Input: part model. Units: mm. Frame: model coordinates. A direction names the side the tool comes from. Give positions to 0.01 mm unless a question says otherwise; leave off trailing zeros. Loops run counter-clockwise (first coordinate to the right, second up) from the corner with the lowest first, then second, coordinate; pieces in that order, holes last. Notation, with made-up numbers: M 31,40 L 64,40 A21 ccw 64,50 Z; hole C 80,-29.5 d2. An arc over 180 degrees is marked long. Use a Markdown table: item, result. Add a question column.
from build123d import *

# Parameters (mm, degrees)
SKETCH1_R               = 1.05
SKETCH1_R_2             = 4.95
BOSS_EXTRUDE1_DEPTH     = 1.5
CIRPATTERN1_COUNT       = 14
SKETCH2_R               = 3.5
SKETCH2_R_2             = 2
SKETCH2_W               = 2
SKETCH2_H               = 4
SKETCH2_W_2             = 4
SKETCH2_H_2             = 2
BOSS_EXTRUDE2_DEPTH     = 7.5
SKETCH3_R               = 2
CUT_EXTRUDE1_DEPTH      = 0.1
SKETCH4_R               = 1
CUT_EXTRUDE2_DEPTH      = 1
CUT_EXTRUDE3_DEPTH      = 1
CUT_EXTRUDE3_DEPTH_BACK = 10


with BuildPart() as part:
    # Sketch1 → Boss-Extrude1 (new body)
    with BuildSketch(Plane(origin=(0, 0, 0), x_dir=(1, 0, 0), z_dir=(0, 1, 0))):
        with Locations((0, 4.95)):
            Circle(SKETCH1_R)
        Circle(SKETCH1_R_2)
    boss_extrude1 = extrude(amount=BOSS_EXTRUDE1_DEPTH)

    # CirPattern1: Boss-Extrude1 ×14 about axis
    cirpattern1_axis = Axis((0, 0, 0), (0, 1, 0))
    for i in range(1, CIRPATTERN1_COUNT):
        add(boss_extrude1.rotate(cirpattern1_axis, i * 360 / CIRPATTERN1_COUNT))

    # Sketch2 → Boss-Extrude2 (add)
    with BuildSketch(Plane(origin=(0, 1.5, 0), x_dir=(1, 0, 0), z_dir=(0, 1, 0))):
        Circle(SKETCH2_R)
        Circle(SKETCH2_R_2, mode=Mode.SUBTRACT)
        Rectangle(SKETCH2_W, SKETCH2_H, mode=Mode.SUBTRACT)
        Rectangle(SKETCH2_W_2, SKETCH2_H_2, mode=Mode.SUBTRACT)
        with BuildLine():
            ThreePointArc((-1, 1.732050808), (-0.517638086, 1.931851654), (9e-09, 2))
            Line((9e-09, 2), (-1, 2))
            Line((-1, 2), (-1, 1.732050808))
        make_face()
        with BuildLine():
            Line((1, 1.732050808), (1, 2))
            Line((1, 2), (9e-09, 2))
            ThreePointArc((9e-09, 2), (0.517638095, 1.931851651), (1, 1.732050808))
        make_face()
        with BuildLine():
            Line((2, 1), (1.732050808, 1))
            ThreePointArc((1.732050808, 1), (1.931851653, 0.51763809), (2, 0))
            Line((2, 0), (2, 1))
        make_face()
        with BuildLine():
            ThreePointArc((1.732050808, 1), (1.414213562, 1.414213562), (1, 1.732050808))
            Line((1, 1.732050808), (1, 1))
            Line((1, 1), (1.732050808, 1))
        make_face()
        with BuildLine():
            Line((-1, 1), (-1, 1.732050808))
            ThreePointArc((-1, 1.732050808), (-1.414213562, 1.414213562), (-1.732050808, 1))
            Line((-1.732050808, 1), (-1, 1))
        make_face()
        with BuildLine():
            ThreePointArc((-2, 0), (-1.931851653, 0.51763809), (-1.732050808, 1))
            Line((-1.732050808, 1), (-2, 1))
            Line((-2, 1), (-2, 0))
        make_face()
        with BuildLine():
            ThreePointArc((-1.732050808, -1), (-1.931851653, -0.51763809), (-2, 0))
            Line((-2, 0), (-2, -1))
            Line((-2, -1), (-1.732050808, -1))
        make_face()
        with BuildLine():
            Line((-1, -1.732050808), (-1, -1))
            Line((-1, -1), (-1.732050808, -1))
            ThreePointArc((-1.732050808, -1), (-1.414213562, -1.414213562), (-1, -1.732050808))
        make_face()
        with BuildLine():
            ThreePointArc((0, -2), (-0.51763809, -1.931851653), (-1, -1.732050808))
            Line((-1, -1.732050808), (-1, -2))
            Line((-1, -2), (0, -2))
        make_face()
        with BuildLine():
            Line((1, -2), (1, -1.732050808))
            ThreePointArc((1, -1.732050808), (0.51763809, -1.931851653), (0, -2))
            Line((0, -2), (1, -2))
        make_face()
        with BuildLine():
            Line((1.732050808, -1), (1, -1))
            Line((1, -1), (1, -1.732050808))
            ThreePointArc((1, -1.732050808), (1.414213562, -1.414213562), (1.732050808, -1))
        make_face()
        with BuildLine():
            Line((2, -1), (2, 0))
            ThreePointArc((2, 0), (1.931851653, -0.51763809), (1.732050808, -1))
            Line((1.732050808, -1), (2, -1))
        make_face()
    extrude(amount=BOSS_EXTRUDE2_DEPTH)

    # Sketch3 → Cut-Extrude1 (cut)
    with BuildSketch(Plane(origin=(0, 9, 0), x_dir=(1, 0, 0), z_dir=(0, 1, 0))):
        Circle(SKETCH3_R)
    extrude(amount=-CUT_EXTRUDE1_DEPTH, mode=Mode.SUBTRACT)

    # Sketch4 → Cut-Extrude2 (cut)
    with BuildSketch(Plane.XZ):
        Circle(SKETCH4_R)
    extrude(amount=-CUT_EXTRUDE2_DEPTH, mode=Mode.SUBTRACT)

    # Sketch5 → Cut-Extrude3 (cut, two sides)
    with BuildSketch(Plane(origin=(0, 9, 0), x_dir=(1, 0, 0), z_dir=(0, 1, 0))) as cut_extrude3_sk:
        with BuildLine():
            Line((-1.594989552, 6), (1.594989552, 6))
            Line((1.594989552, 6), (0.653815854, 3.43838986))
            ThreePointArc((0.653815854, 3.43838986), (0, 3.5), (-0.653815854, 3.43838986))
            Line((-0.653815854, 3.43838986), (-1.594989552, 6))
        make_face()
        with BuildLine():
            Line((1.594989552, -6), (0.653815854, -3.43838986))
            ThreePointArc((0.653815854, -3.43838986), (0, -3.5), (-0.653815854, -3.43838986))
            Line((-0.653815854, -3.43838986), (-1.594989552, -6))
            Line((-1.594989552, -6), (1.594989552, -6))
        make_face()
    extrude(amount=CUT_EXTRUDE3_DEPTH, mode=Mode.SUBTRACT)
    extrude(cut_extrude3_sk.sketch, amount=-CUT_EXTRUDE3_DEPTH_BACK, mode=Mode.SUBTRACT)


solid = part.part
1) Ray query, line 1 (Z direction, x = 0, y = 0.5); line 2 (Y direction, x = 2, z = -3.5); line 3 (Z direction, x = 0.5, y = 3). Return the intervals inside material, ascending. Write a range as [from, to].
2) Section query D-D, the plane x = 1.5. Return the cut outline in (y, z), and give its area (3 significant figures).
3) Pull-direction query (Z, two-part tool) for faces 1 (the flat face through (-0.903, 0.761, -4.116)), 2 (the cylindrical face through (5.855, 0.74, -1.311)), 3 (the flat face through (0.91, 0.76, 4.14)); classes: pulls with the +Z half, pulls with the -Z half, needs draft (parallel to the pull), parting line crosses it, or undercut.
4) Section query A-A, the plane y = 4. Return the cut outline in (x, z), and give its area (3 significant figures).
5) Section query C-C, the plane z = 2.5. Return the cut outline in (x, y), and give its area (3 significant figures).
6) Contact query for flat-ended pins moving along their axis: P1, Ø1.6, axis at x = 4, z = 0.5, coming from the +Y side; P2, Ø3, axis at y = 2.5, z = 2.5, coming from the +X side; P3, Ø0.8, axis at x = 1.5, y = 7, coming from the -Z side; P4, Ø2, axis at x = 2.5, y = 5.5, coming from the -Z side. Output: stop coordinate, or through.
7) Section query B-B, the plane x = -4.75. Return the cut outline in (y, z).
8) Reachability of faces 4 (the flat face through (-4, 1.5, 0)), 5 (the flat face through (-0.903, 0.761, 4.116)), 6 (the flat face through (0.91, 0.76, -4.14)), 7 (the flat face through (0, 1, 0)) from +Z, -Z, +X, -X, +Y, -Y: full face, straight path, thin tool, end or side. Return the list, or none.
Entries:
| question | item | result |
|---|---|---|
| 1 | line 1 | z = [-3.5, -1], [1, 3.5] |
| 1 | line 2 | y = [0, 1.5] |
| 1 | line 3 | z = [-3.46, -1.94], [1.94, 3.46] |
| 2 | outline | M 0,-5.29 L 1.5,-5.29 L 1.5,-3.16 L 9,-3.16 L 9,-1.32 L 8.9,-1.32 L 8.9,-1 L 1.5,-1 L 1.5,1 L 8.9,1 L 8.9,1.32 L 9,1.32 L 9,3.16 L 1.5,3.16 L 1.5,5.29 L 0,5.29 Z |
| 2 | area | 48.2 mm² |
| 3 | face 1 | pulls with the -Z half |
| 3 | face 2 | undercut |
| 3 | face 3 | pulls with the +Z half |
| 4 | outline | C 0,0 d7; hole M -1.73,-1 L -1,-1 L -1,-1.73 A2 ccw 1,-1.73 L 1,-1 L 1.73,-1 A2 ccw 1.73,1 L 1,1 L 1,1.73 A2 ccw -1,1.73 L -1,1 L -1.73,1 A2 ccw Z |
| 4 | area | 27.2 mm² |
| 5 | outline | M -4.74,0 L 4.74,0 L 4.74,1.5 L 2.45,1.5 L 2.45,9 L -2.45,9 L -2.45,1.5 L -4.74,1.5 Z |
| 5 | area | 51.0 mm² |
| 6 | P1 | stops at y = 9 |
| 6 | P2 | stops at x = 5.84 |
| 6 | P3 | stops at z = -3.32 |
| 6 | P4 | stops at z = -3.16 |
| 7 | outline | M 0,-3.66 L 1.5,-3.66 L 1.5,-2.51 L 0,-2.51 Z; M 0,-2.15 L 1.5,-2.15 L 1.5,2.15 L 0,2.15 Z; M 0,2.51 L 1.5,2.51 L 1.5,3.66 L 0,3.66 Z |
| 8 | face 4 | -X, +Y |
| 8 | face 5 | +Z, +Y, -Y |
| 8 | face 6 | -Z, +Y, -Y |
| 8 | face 7 | -Y |
